```python
from build123d import *

# Parameters (mm, degrees)
F0_W           = 5
F0_H           = 5
F1_DEPTH       = 200
F3_DEPTH       = 1.2
F5_D           = 4
F5_CSINK_D     = 8.7
F5_CSINK_ANGLE = 90
F6_DEPTH       = 170
F8_DEPTH       = 25


with BuildPart() as f1:
    # F0 (on Right) → F1 (new body)
    with BuildSketch(Plane.YZ):
        Polygon((0, 30), (0, 15), (6.1031254008, 15), (10, 15), (10, 25), (15, 25), (20, 25), (20, 30), align=None)
        with Locations((17.5, 22.5)):
            Rectangle(F0_W, F0_H)
        with Locations((17.5, 7.5)):
            Rectangle(F0_W, F0_H)
        Polygon((0, 15), (0, 0), (20, 0), (20, 5), (15, 5), (10, 5), (10, 15), (6.1031254008, 15), align=None)
    extrude(amount=F1_DEPTH)

    # F2 (on face) → F3 (join)
    with BuildSketch(Plane.YZ.offset(200)):
        Polygon((20, 30), (0, 30), (0, 0), (20, 0), (20, 10), (15, 10), (15, 5), (10, 5), (10, 25), (15, 25), (15, 20), (20, 20), align=None)
        Polygon((20, 10), (20, 20), (15, 20), (15, 25), (10, 25), (10, 5), (15, 5), (15, 10), align=None)
    extrude(amount=F3_DEPTH)

    # F5 (through all)
    with Locations(Plane(origin=(0, 10, 0), x_dir=(-1, 0, 0), z_dir=(0, 1, 0))):
        with Locations((-15, 15), (-185, 15), (-100, 15)):
            CounterSinkHole(F5_D / 2, F5_CSINK_D / 2, counter_sink_angle=F5_CSINK_ANGLE)

    # F6 (cut): a face of the model
    f6_faces = [f1.faces().sort_by_distance(p)[0] for p in [
        (201.2, 10, 15),
    ]]
    extrude(f6_faces, amount=-F6_DEPTH, mode=Mode.SUBTRACT)

    # F7 (on face) → F8 (cut)
    with BuildSketch(Plane(origin=(0, 10, 0), x_dir=(-1, 0, 0), z_dir=(0, 1, 0))):
        with BuildLine():
            ThreePointArc((-27.85, 15), (-26.2, 13.35), (-24.55, 15))
            ThreePointArc((-24.55, 15), (-26.2, 16.65), (-27.85, 15))
        make_face()
        with BuildLine():
            ThreePointArc((-24.55, 15), (-26.2, 16.65), (-27.85, 15))
            ThreePointArc((-27.85, 15), (-26.2, 13.35), (-24.55, 15))
        make_face()
    extrude(amount=-F8_DEPTH, mode=Mode.SUBTRACT)


solid = f1.part
```
Could you check a few things on this model? Use its own coordinates, in mm. A direction names the side the tool comes from. Give positions to 0.01 mm unless a question says otherwise; leave off trailing zeros. Order: outer loops, then holes, each group sorted by start corner. A loop starts at its lowest first (then second) coordinate and runs counter-clockwise, first axis right, second up.
Q1. Suppose I cut it at B-B, the plane y = 12. Write out the boundary of the cut face in (x, z), and give its area (3 significant figures).
Q2. We'd pull the mould along Z, two halves only. Please class faces 4 (the flat face through (15, 20, 5)), 5 (the flat face through (15, 10, 30)), 6 (the flat face through (15, 12, 25)), 7 (the flat face through (18.85, 10, 12.64)): +Z half, -Z half, draft (parallel to the pull), parting line (faces both ways), or undercut.
Q3. Suppose I cut it at D-D, the plane x = 5. Write out the boundary of the cut face in (y, z), and give its area (3 significant figures).
Q4. Suppose I cut it at C-C, the plane z = 15. Write out the boundary of the cut face in (x, y).
Q5. I'm going to push flat-ended pins straight in: P1, Ø4, axis at x = 26.2, z = 15, coming from the -Y side; P2, Ø6, axis at x = 8, z = 16, coming from the +Y side. Where does each tip first touch, or does it pass through?
Q6. Suppose I cut it at A-A, the plane x = 15. Write out the boundary of the cut face in (y, z).
Q7. If I drill on line 1 along X through (y, z) = (4, 15); line 2 along Z through (x, y) = (14, 11.5); line 3 along Z through (x, y) = (26.2, 4.75), over which ranges is the centre line in solid material (lowest first)?
Q8. For faces 1 (the flat face through (12, 0, 15)), 2 (the flat face through (15, 15, 22)), 3 (the flat face through (15, 17, 10)), which set-ups out of +Z, -Z, +X, -X, +Y, -Y let a thin tool reach every point of the face, with its end or its side?
Solution:
1. outline: (0, 0) - (31.2, 0) - (31.2, 5) - (0, 5) - close; (0, 25) - (31.2, 25) - (31.2, 30) - (0, 30) - close
1. area: 312 mm2
2. face 4: draft
2. face 5: +Z half
2. face 6: undercut
2. face 7: undercut
3. outline: (0, 0) - (20, 0) - (20, 10) - (15, 10) - (15, 5) - (10, 5) - (10, 25) - (15, 25) - (15, 20) - (20, 20) - (20, 30) - (0, 30) - close
3. area: 450 mm2
4. outline: (0, 0) - (13, 0) - (13, 7.65) - (10.65, 10) - (0, 10) - close; (17, 0) - (24.55, 0) - (24.55, 10) - (19.35, 10) - (17, 7.65) - close; (27.85, 0) - (31.2, 0) - (31.2, 10) - (27.85, 10) - close
5. P1: stops at y = 0
5. P2: stops at y = 10
6. outline: (0, 0) - (20, 0) - (20, 10) - (15, 10) - (15, 5) - (10, 5) - (10, 10.65) - (7.65, 13) - (0, 13) - close; (0, 17) - (7.65, 17) - (10, 19.35) - (10, 25) - (15, 25) - (15, 20) - (20, 20) - (20, 30) - (0, 30) - close
7. line 1: x = 0 to 13, 17 to 24.55, 27.85 to 31.2
7. line 2: z = 0 to 5, 25 to 30
7. line 3: z = 0 to 13.35, 16.65 to 30
8. face 1: +Z, -Z, +X, -X, -Y
8. face 2: +X, -X
8. face 3: +X, -X, +Y
